Verification items for the finished model (mm, model axes). A direction names the side the tool comes from. Round coordinates to 2 decimals unless told otherwise and drop trailing zeros. Write each loop counter-clockwise with the first axis right and the second up, starting at its lowest first coordinate (ties: lowest second). Pieces come first, ordered by that corner, then holes. Notation, with made-up numbers: (-22, 44) - (-1, 44) arc R24 cw to (-1, 58) - close; hole circle Ø2 at (32, 61). An arc over 180 degrees is marked (long way). Answer as a JSON object with one key per item and string values.
```python
from build123d import *

# Parameters (mm, degrees)
F1_DEPTH = 20
F2_R     = 5
F3_R     = 10
F4_DEPTH = 20.001
F5_W     = 20
F5_H     = 5
F6_DEPTH = 15


with BuildPart() as f1:
    # F0 (on Front) → F1 (new body)
    with BuildSketch(Plane.XZ):
        Polygon((0, 39.944667), (0, 0), (111.015879, 0), (111.015879, 14.474314), (67.249916, 14.474314), (67.249916, 39.944667), align=None)
    extrude(amount=F1_DEPTH)

    # F2
    f2_edges = [f1.edges().sort_by_distance(p)[0] for p in [
        (67.249916, -10, 39.944667),
        (111.015879, -10, 14.474314),
        (0, -10, 39.944667),
    ]]
    fillet(f2_edges, radius=F2_R)

    # F3 (on face) → F4 (cut, through all)
    with BuildSketch(Plane.XZ.offset(20)):
        with Locations((30, 14.474314)):
            Circle(F3_R)
    extrude(amount=-F4_DEPTH, mode=Mode.SUBTRACT)

    # F5 (on face) → F6 (cut)
    with BuildSketch(Plane.XZ.offset(20)):
        with Locations((81.015879, 2.5)):
            Rectangle(F5_W, F5_H)
    extrude(amount=-F6_DEPTH, mode=Mode.SUBTRACT)


solid = f1.part
```
Q1. Set-up check for faces 4 (the flat face through (81, -5, 3)), 5 (the cylindrical face through (109.59, -10.14, 12.97)): record each of +Z, -Z, +X, -X, +Y, -Y from which the full face is reachable in a straight line by a thin tool's end or side.
Geometry check:
{"face 4": "-Z, -Y", "face 5": "+Z, +X, +Y, -Y"}
Q2. Section check A-A, the plane x = 30. Record the cut outline in (y, z).
Geometry check:
{"outline": "(-20, 0) - (0, 0) - (0, 4.47) - (-20, 4.47) - close; (-20, 24.47) - (0, 24.47) - (0, 39.94) - (-20, 39.94) - close"}
Q3. Section check C-C, the plane z = 23.5. Record the cut outline in (x, y), then the cut area to 3 significant figures.
Geometry check:
{"outline": "(0, -20) - (25.69, -20) - (25.69, 0) - (0, 0) - close; (34.31, -20) - (67.25, -20) - (67.25, 0) - (34.31, 0) - close", "area": "1,170 mm2"}
Q4. Section check B-B, the plane y = -9.75. Record the cut outline in (x, z), then the cut area to 3 significant figures.
Geometry check:
{"outline": "(0, 0) - (71.02, 0) - (71.02, 5) - (91.02, 5) - (91.02, 0) - (111.02, 0) - (111.02, 9.47) arc R5 ccw to (106.02, 14.47) - (67.25, 14.47) - (67.25, 34.94) arc R5 ccw to (62.25, 39.94) - (5, 39.94) arc R5 ccw to (0, 34.94) - close; hole circle Ø20 at (30, 14.47)", "area": "2,890 mm2"}
Q5. Gauge pin test, flat ends, axial feed: P1, Ø10, axis at x = 93.5, y = -6.5, coming from the +Z side; P2, Ø4, axis at x = 83, z = 2.5, coming from the -Y side; P3, Ø6, axis at x = 38.5, y = -13.5, coming from the -Z side. Record the tip position at first contact, or that the pin passes through.
Geometry check:
{"P1": "stops at z = 14.47", "P2": "stops at y = -5", "P3": "stops at z = 0"}
Q6. Release check for a two-part mould opening along X. For faces 1 (the flat face through (87, -10, 14.474)), 2 (the flat face through (67.25, -10, 25)), 3 (the flat face through (91.016, -13, 2)) record: released by +X, released by -X, zero draft, split by the parting line, or undercut.
Geometry check:
{"face 1": "zero draft", "face 2": "released by +X", "face 3": "undercut"}
Q7. Section check D-D, the plane y = -3.75. Record the cut outline in (x, z), then the cut area to 3 significant figures.
Geometry check:
{"outline": "(0, 0) - (111.02, 0) - (111.02, 9.47) arc R5 ccw to (106.02, 14.47) - (67.25, 14.47) - (67.25, 34.94) arc R5 ccw to (62.25, 39.94) - (5, 39.94) arc R5 ccw to (0, 34.94) - close; hole circle Ø20 at (30, 14.47)", "area": "2,990 mm2"}
Q8. Material ranges on line 1 along Z through (x, y) = (30, -15.75); line 2 along X through (y, z) = (-9.5, 2); line 3 along X through (y, z) = (-12.75, 15), recorded low to high. Write a range as [from, to].
Geometry check:
{"line 1": "z = [0, 4.47], [24.47, 39.94]", "line 2": "x = [0, 71.02], [91.02, 111.02]", "line 3": "x = [0, 20.01], [39.99, 67.25]"}
